from build123d import *

# Parameters (mm, degrees)
BOSS_EXTRUDE1_DEPTH              = 320.675
BOSS_EXTRUDE1_DEPTH_BACK         = 320.675
SKETCH3_W                        = 50.8
SKETCH3_H                        = 25.4
SKETCH3_W_2                      = 44.45
SKETCH3_H_2                      = 19.05
CUT_EXTRUDE1_DEPTH               = 323.680609311
CUT_EXTRUDE1_DEPTH_BACK          = 323.680609311
SKETCH8_R                        = 14.2875
CUT_EXTRUDE2_DEPTH               = 323.680609311
F_10_CLEARANCE_HOLE1_D           = 4.9784
F_10_CLEARANCE_HOLE1_DEPTH       = 5.08
F_10_CLEARANCE_HOLE1_TIP         = 1.495662253
F_10_CLEARANCE_HOLE2_D           = 4.9784
F_10_CLEARANCE_HOLE3_D           = 4.9784
F_10_CLEARANCE_HOLE4_D           = 4.9784
F_10_CLEARANCE_HOLE4_DEPTH       = 5.08
F_10_CLEARANCE_HOLE4_TIP         = 1.495662253
F_10_CLEARANCE_HOLE5_D           = 4.9784
TAP_DRILL_FOR_8_32_TAP1_D        = 3.4544
F_10_CLEARANCE_HOLE6_AT_2_COUNT  = 2
F_10_CLEARANCE_HOLE6_AT_2_PITCH  = 21.6408
F_10_CLEARANCE_HOLE6_AT_3_COUNT  = 2
F_10_CLEARANCE_HOLE6_AT_3_PITCH  = 32.224022105
F_10_CLEARANCE_HOLE6_AT_4_COUNT  = 2
F_10_CLEARANCE_HOLE6_AT_4_PITCH  = 23.876
F_10_CLEARANCE_HOLE6_AT_5_COUNT  = 2
F_10_CLEARANCE_HOLE6_AT_5_PITCH  = 269.79183685
F_10_CLEARANCE_HOLE6_AT_6_COUNT  = 2
F_10_CLEARANCE_HOLE6_AT_6_PITCH  = 268.9225
F_10_CLEARANCE_HOLE6_AT_7_COUNT  = 2
F_10_CLEARANCE_HOLE6_AT_7_PITCH  = 292.7985
F_10_CLEARANCE_HOLE6_AT_8_COUNT  = 2
F_10_CLEARANCE_HOLE6_AT_8_PITCH  = 293.597148874
F_10_0_1935_DIAMETER_HOLE1_D     = 4.9149
F_10_0_1935_DIAMETER_HOLE1_DEPTH = 3.302
F_10_0_1935_DIAMETER_HOLE1_TIP   = 1.476584928
CUT_EXTRUDE4_DEPTH               = 5.08
F_1_4_0_25_DIAMETER_HOLE1_D      = 6.35


with BuildPart() as part:
    # Sketch3 → Boss-Extrude1 (new, two sides: drawn at the far end of the back side and taken through both)
    with BuildSketch(Plane.XY.offset(-BOSS_EXTRUDE1_DEPTH_BACK)):
        Rectangle(SKETCH3_W, SKETCH3_H)
        Rectangle(SKETCH3_W_2, SKETCH3_H_2, mode=Mode.SUBTRACT)
    extrude(amount=BOSS_EXTRUDE1_DEPTH + BOSS_EXTRUDE1_DEPTH_BACK)

    # Sketch4 → Cut-Extrude1 (cut, two sides: drawn at the far end of the back side and taken through both)
    with BuildSketch(Plane(origin=(0, 12.7, 0), x_dir=(1, 0, 0), z_dir=(0, 1, 0)).offset(-CUT_EXTRUDE1_DEPTH_BACK)):
        Polygon((1322.117470931, -320.675), (25.4, -320.675), (-25.4, -320.675), (25.4, -305.627354456), (1268.718301677, 62.660305034), (3837.350959621, 420.474595165), (3890.750128875, 37.139290131), align=None)
    extrude(amount=CUT_EXTRUDE1_DEPTH + CUT_EXTRUDE1_DEPTH_BACK, mode=Mode.SUBTRACT)

    # Sketch8 → Cut-Extrude2 (cut, through all)
    with BuildSketch(Plane(origin=(0, 12.7, 0), x_dir=(1, 0, 0), z_dir=(0, 1, 0))):
        with Locations(Location((0, 266.954, 0), (0, 0, 180))):
            Circle(SKETCH8_R)
    extrude(amount=-CUT_EXTRUDE2_DEPTH, mode=Mode.SUBTRACT)

    # #10 Clearance Hole1
    with Locations(Plane(origin=(0, -12.7, 0), x_dir=(-1, 0, 0), z_dir=(0, -1, 0))):
        with Locations((-12.6238, -284.753033923), (12.7762, -284.753033923), (12.7762, -301.263033923), (-12.6238, -301.263033923)):
            Hole(F_10_CLEARANCE_HOLE1_D / 2, depth=F_10_CLEARANCE_HOLE1_DEPTH)
            with Locations((0, 0, -(F_10_CLEARANCE_HOLE1_DEPTH + F_10_CLEARANCE_HOLE1_TIP / 2))):  # 118° drill point
                Cone(0, F_10_CLEARANCE_HOLE1_D / 2, F_10_CLEARANCE_HOLE1_TIP, mode=Mode.SUBTRACT)

    # #10 Clearance Hole2 (through all)
    with Locations(Plane(origin=(25.4, 0, 0), x_dir=(0, 0, -1), z_dir=(1, 0, 0))):
        with Locations((314.325, 6.35), (295.275, 6.35)):
            Hole(F_10_CLEARANCE_HOLE2_D / 2)

    # #10 Clearance Hole3 (through all)
    with Locations(Plane(origin=(25.4, 0, 0), x_dir=(0, 0, -1), z_dir=(1, 0, 0))):
        with Locations((105.029, 6.35), (79.629, 6.35), (54.229, 6.35), (28.829, 6.35), (3.429, 6.35), (-289.126683504, 6.388229415), (-263.726683504, 6.388229415), (-238.326683504, 6.388229415)):
            Hole(F_10_CLEARANCE_HOLE3_D / 2)

    # #10 Clearance Hole4
    with Locations(Plane(origin=(0, 12.7, 0), x_dir=(1, 0, 0), z_dir=(0, 1, 0))):
        with Locations((17.786, 281.371028265), (-17.786, 252.536971735)):
            Hole(F_10_CLEARANCE_HOLE4_D / 2, depth=F_10_CLEARANCE_HOLE4_DEPTH)
            with Locations((0, 0, -(F_10_CLEARANCE_HOLE4_DEPTH + F_10_CLEARANCE_HOLE4_TIP / 2))):  # 118° drill point
                Cone(0, F_10_CLEARANCE_HOLE4_D / 2, F_10_CLEARANCE_HOLE4_TIP, mode=Mode.SUBTRACT)

    # #10 Clearance Hole5 (through all)
    with Locations(Plane(origin=(0, 12.7, 0), x_dir=(1, 0, 0), z_dir=(0, 1, 0))):
        with Locations((-0.0762, -211.551177228)):
            Hole(F_10_CLEARANCE_HOLE5_D / 2)

    # Tap Drill for #8-32 Tap1 (through all)
    with Locations(Plane(origin=(0, 12.7, 0), x_dir=(1, 0, 0), z_dir=(0, 1, 0))):
        with Locations((11.355922339, 252.94442528)):
            Hole(TAP_DRILL_FOR_8_32_TAP1_D / 2)

    # Sketch27 → #10 Clearance Hole6 (revolve, cut)
    with BuildSketch(Plane(origin=(-9.795655012, 12.7, -238.47425), x_dir=(0, 0, 1), z_dir=(1, 0, 0))):
        Polygon((0, 0), (0, 25.4), (5.2197, 25.4), (2.4892, 22.258919064), (2.4892, 0), align=None)
    f_10_clearance_hole6 = revolve(axis=Axis((-9.795655012, 19.05, -238.47425), (0, -1, 0)), mode=Mode.SUBTRACT)

    # #10 Clearance Hole6 at 2: #10 Clearance Hole6 ×2
    with Locations(*[(i * F_10_CLEARANCE_HOLE6_AT_2_PITCH, 0, 0) for i in range(1, F_10_CLEARANCE_HOLE6_AT_2_COUNT)]):
        add(f_10_clearance_hole6, mode=Mode.SUBTRACT)

    # #10 Clearance Hole6 at 3: #10 Clearance Hole6 ×2
    with Locations(*[Vector(0.6715735214342003, 0, 0.7409379227090943) * (i * F_10_CLEARANCE_HOLE6_AT_3_PITCH) for i in range(1, F_10_CLEARANCE_HOLE6_AT_3_COUNT)]):
        add(f_10_clearance_hole6, mode=Mode.SUBTRACT)

    # #10 Clearance Hole6 at 4: #10 Clearance Hole6 ×2
    with Locations(*[(0, 0, i * F_10_CLEARANCE_HOLE6_AT_4_PITCH) for i in range(1, F_10_CLEARANCE_HOLE6_AT_4_COUNT)]):
        add(f_10_clearance_hole6, mode=Mode.SUBTRACT)

    # #10 Clearance Hole6 at 5: #10 Clearance Hole6 ×2
    with Locations(*[Vector(0.08021295326304838, 0, 0.9967777496156403) * (i * F_10_CLEARANCE_HOLE6_AT_5_PITCH) for i in range(1, F_10_CLEARANCE_HOLE6_AT_5_COUNT)]):
        add(f_10_clearance_hole6, mode=Mode.SUBTRACT)

    # #10 Clearance Hole6 at 6: #10 Clearance Hole6 ×2
    with Locations(*[(0, 0, i * F_10_CLEARANCE_HOLE6_AT_6_PITCH) for i in range(1, F_10_CLEARANCE_HOLE6_AT_6_COUNT)]):
        add(f_10_clearance_hole6, mode=Mode.SUBTRACT)

    # #10 Clearance Hole6 at 7: #10 Clearance Hole6 ×2
    with Locations(*[(0, 0, i * F_10_CLEARANCE_HOLE6_AT_7_PITCH) for i in range(1, F_10_CLEARANCE_HOLE6_AT_7_COUNT)]):
        add(f_10_clearance_hole6, mode=Mode.SUBTRACT)

    # #10 Clearance Hole6 at 8: #10 Clearance Hole6 ×2
    with Locations(*[Vector(0.07370916265026073, 0, 0.9972797798719262) * (i * F_10_CLEARANCE_HOLE6_AT_8_PITCH) for i in range(1, F_10_CLEARANCE_HOLE6_AT_8_COUNT)]):
        add(f_10_clearance_hole6, mode=Mode.SUBTRACT)

    # #10 (0.1935) Diameter Hole1
    with Locations(Plane(origin=(25.4, 0, 0), x_dir=(0, 0, -1), z_dir=(1, 0, 0))):
        with Locations((269.875, 6.35)):
            Hole(F_10_0_1935_DIAMETER_HOLE1_D / 2, depth=F_10_0_1935_DIAMETER_HOLE1_DEPTH)
            with Locations((0, 0, -(F_10_0_1935_DIAMETER_HOLE1_DEPTH + F_10_0_1935_DIAMETER_HOLE1_TIP / 2))):  # 118° drill point
                Cone(0, F_10_0_1935_DIAMETER_HOLE1_D / 2, F_10_0_1935_DIAMETER_HOLE1_TIP, mode=Mode.SUBTRACT)

    # Sketch30 → Cut-Extrude4 (cut)
    with BuildSketch(Plane(origin=(0, -12.7, 0), x_dir=(1, 0, 0), z_dir=(0, 1, 0))):
        with BuildLine():
            Line((-17.533651131, -318.344881309), (-5.356640498, -314.737886431))
            Line((-5.356640498, -314.737886431), (-6.078039474, -312.302484305))
            ThreePointArc((-6.078039474, -312.302484305), (-13.970042229, -308.017476427), (-18.255050107, -315.909479182))
            Line((-18.255050107, -315.909479182), (-17.533651131, -318.344881309))
        make_face()
    extrude(amount=CUT_EXTRUDE4_DEPTH, mode=Mode.SUBTRACT)

    # 1/4 (0.25) Diameter Hole1 (through all)
    with Locations(Plane(origin=(0, 12.7, 0), x_dir=(1, 0, 0), z_dir=(0, 1, 0))):
        with Locations((0, -71.851177228), (0, -249.651177228), (0, 182.148822772)):
            Hole(F_1_4_0_25_DIAMETER_HOLE1_D / 2)


solid = part.part
The model under review builds one solid part; all positions refer to its coordinate system, in mm. A direction names the side the tool comes from. Give positions to 0.01 mm unless a question says otherwise; leave off trailing zeros. Write each loop counter-clockwise with the first axis right and the second up, starting at its lowest first coordinate (ties: lowest second). Pieces come first, ordered by that corner, then holes.
1. Add section B-B, the plane z = 197.5. Write out the cut boundary in (x, y) (3 decimals), plus the area to 3 significant figures.
2. For P1, Ø8, axis at x = 11.85, z = 30.45, coming from the -Y side; P2, Ø4.5, axis at x = 11.85, z = -238.47, coming from the +Y side; P3, Ø4, axis at y = 6.35, z = -269.875, coming from the +X side (3 decimals); P4, Ø2, axis at x = 11, y = 10, coming from the +Z side, all flat-tipped, find the tip position at first contact; note any pin that passes through.
3. Draft analysis for pull direction Y (two halves, no side actions). For faces 1 (the cylindrical face through (-6.59, -11.09, -279.63)), 2 (the conical face through (-9.911, -9.711, -217.217)), 3 (the flat face through (-22.225, 0, -5)), state which applies: +Y half, -Y half, draft (parallel to the pull), parting line (faces both ways), or undercut.
4. Tool access review of faces 4 (the flat face through (0, 9.525, -5)), 5 (the conical face through (-12.01, -9.71, 55.73)): name each direction out of +Z, -Z, +X, -X, +Y, -Y from which nothing blocks a thin tool from reaching the whole face with its end or side.
5. Wall thickness on L1, parallel to X at y = -9, z = -4 (3 decimals); L2, parallel to Y at x = 14, z = 191.5 (3 decimals); L3, parallel to Y at x = 17, z = -280 (3 decimals): over which ranges is each line inside the solid? List them lowest first.
6. Add section A-A, the plane y = -1.5. Write out the cut boundary in (x, z) (3 decimals).
Worked answers:
1. outline: (-25.4, -12.7) - (25.4, -12.7) - (25.4, 12.7) - (-25.4, 12.7) - close; hole (-22.225, -9.525) - (22.225, -9.525) - (22.225, 9.525) - (-22.225, 9.525) - close
1. area: 444 mm2
2. P1: stops at y = -11.3
2. P2: passes through
2. P3: stops at x = -22.225
2. P4: stops at z = 310.19
3. face 1: draft
3. face 2: -Y half
3. face 3: undercut
4. face 4: +Z, -Z
4. face 5: -Y
5. L1: x = -25.4 to -22.225, 22.225 to 25.4
5. L2: y = -12.7 to -9.525, 9.525 to 12.7
5. L3: y = -12.7 to -9.525
6. outline: (-25.4, -320.675) - (-22.225, -320.675) - (-22.225, 319.735) - (-25.4, 320.675) - close; (22.225, -320.675) - (25.4, -320.675) - (25.4, 305.627) - (22.225, 306.568) - close
